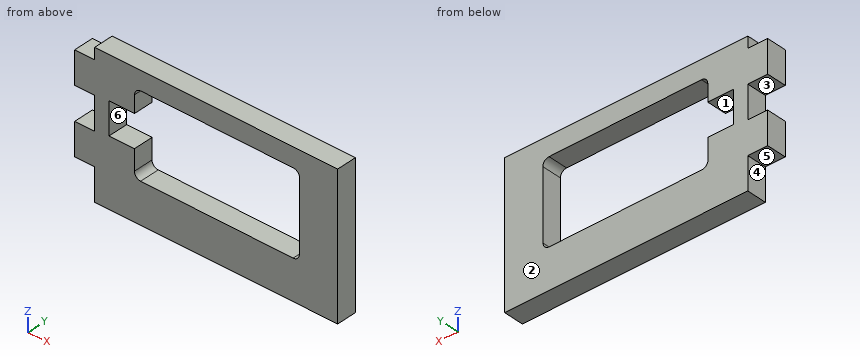
```python
from build123d import *

# Parameters (mm, degrees)
SKETCH1_W           = 127
SKETCH1_H           = 101.6
BOSS_EXTRUDE1_DEPTH = 4.800000052
CUT_EXTRUDE1_DEPTH  = 163.710171779
SKETCH4_W           = 127
SKETCH4_H           = 101.6
SKETCH4_W_2         = 63.302571571
SKETCH4_H_2         = 39.058596
CUT_EXTRUDE3_DEPTH  = 163.710171779
SKETCH5_W           = 4.800000052
SKETCH5_H           = 7.8117192
SKETCH5_H_2         = 7.874
SKETCH5_H_3         = 7.7494384
CUT_EXTRUDE4_DEPTH  = 133.639014141
SKETCH6_W           = 6.142649692
SKETCH6_H           = 7.722699729
CUT_EXTRUDE5_DEPTH  = 133.639014141
SKETCH7_W           = 58.502571519
SKETCH7_H           = 5.08
CUT_EXTRUDE6_DEPTH  = 133.639014141


with BuildPart() as part:
    # Sketch1 → Boss-Extrude1 (new body)
    with BuildSketch(Plane(origin=(0, 0, 0), x_dir=(1, 0, 0), z_dir=(0, 1, 0))):
        with Locations((63.5, 50.8)):
            Rectangle(SKETCH1_W, SKETCH1_H)
    extrude(amount=BOSS_EXTRUDE1_DEPTH)

    # Sketch3 → Cut-Extrude1 (cut, through all)
    with BuildSketch(Plane(origin=(0, 4.800000052, 0), x_dir=(1, 0, 0), z_dir=(0, 1, 0))):
        with BuildLine():
            Line((62.069935242, 45.315244869), (98.769812683, 45.432826029))
            ThreePointArc((98.769812683, 45.432826029), (99.829038472, 45.875546579), (100.264962787, 46.93758742))
            Line((100.264962787, 46.93758742), (100.211138047, 63.737569431))
            ThreePointArc((100.211138047, 63.737569431), (99.768417497, 64.79679522), (98.706376655, 65.232719535))
            Line((98.706376655, 65.232719535), (62.006499215, 65.115138375))
            ThreePointArc((62.006499215, 65.115138375), (60.947273426, 64.672417825), (60.51134911, 63.610376984))
            Line((60.51134911, 63.610376984), (60.565173851, 46.810394973))
            ThreePointArc((60.565173851, 46.810394973), (61.007894401, 45.751169184), (62.069935242, 45.315244869))
        make_face()
    extrude(amount=-CUT_EXTRUDE1_DEPTH, mode=Mode.SUBTRACT)

    # Sketch4 → Cut-Extrude3 (cut, through all)
    with BuildSketch(Plane.XZ):
        with Locations((63.5, -50.8)):
            Rectangle(SKETCH4_W, SKETCH4_H)
        with Locations((77.789401758, -55.255753861)):
            Rectangle(SKETCH4_W_2, SKETCH4_H_2, mode=Mode.SUBTRACT)
    extrude(amount=-CUT_EXTRUDE3_DEPTH, mode=Mode.SUBTRACT)

    # Sketch5 → Cut-Extrude4 (cut, through all)
    with BuildSketch(Plane.XZ):
        with Locations((48.538115998, -39.632315461)):
            Rectangle(SKETCH5_W, SKETCH5_H)
        with Locations((48.538115998, -55.286894261)):
            Rectangle(SKETCH5_W, SKETCH5_H_2)
        with Locations((48.538115998, -70.910332661)):
            Rectangle(SKETCH5_W, SKETCH5_H_3)
    extrude(amount=-CUT_EXTRUDE4_DEPTH, mode=Mode.SUBTRACT)

    # Sketch6 → Cut-Extrude5 (cut, through all)
    with BuildSketch(Plane.XZ):
        with Locations((57.480654221, -54.790150784)):
            Rectangle(SKETCH6_W, SKETCH6_H)
    extrude(amount=-CUT_EXTRUDE5_DEPTH, mode=Mode.SUBTRACT)

    # Sketch7 → Cut-Extrude6 (cut, through all)
    with BuildSketch(Plane(origin=(0, 4.800000052, 0), x_dir=(1, 0, 0), z_dir=(0, 1, 0))):
        with Locations((80.189401784, 38.266455861)):
            Rectangle(SKETCH7_W, SKETCH7_H)
    extrude(amount=-CUT_EXTRUDE6_DEPTH, mode=Mode.SUBTRACT)


solid = part.part
```
Geometry check sheet. Reference: the model listing, model coordinates, mm. Face numbers are marked on the shaded views. A direction names the side the tool comes from. Round coordinates to 2 decimals unless told otherwise and drop trailing zeros. Loops run counter-clockwise (first coordinate to the right, second up) from the corner with the lowest first, then second, coordinate; pieces in that order, holes last. Notation, with made-up numbers: M -13.75,-33 L 36.25,-33 A34 ccw 36.25,6 Z; hole C 28.5,-27 d11. An arc over 180 degrees is marked long. Return JSON: item names as keys, results as strings. Group by question number.
(1) Scan lines: line 1 along X through (y, z) = (0.35, -60); line 2 along X through (y, z) = (0.35, -49); line 3 along Z through (x, y) = (66, 4.15). Record each from-to range of solid material in increasing order. Write a range as [from, to].
(2) Section check C-C, the plane x = 74.5. Enter the section's corners in (y, z).
(3) Section check B-B, the plane z = -58. Enter the section's corners in (x, y).
(4) Go/stop test with a flat-tipped pin: pin 1 (1.4 mm diameter, centred on y = 3.5, z = -57.5, fed in from -X). Record where the tip stops, or that it passes through.
(5) Set-up check for the marked faces 1, 2 and 3: record each of +Z, -Z, +X, -X, +Y, -Y from which the full face is reachable in a straight line by a thin tool's end or side.
(6) Section check D-D, the plane z = -69. Enter the section's corners in (x, y), and give its area (3 significant figures).
(7) Section check A-A, the plane y = 3.25. Enter the section's corners in (x, z), and give its area (3 significant figures).
(8) Mould release check, pull along Z, two halves, no side actions. Record for the marked faces 4, 5 and 6: pulls with the +Z half, pulls with the -Z half, needs draft (parallel to the pull), parting line crosses it, or undercut.
Data:
{
 "1": {"line 1": "[46.14, 60.52], [100.22, 109.44]", "line 2": "[46.14, 60.56], [100.26, 109.44]", "line 3": "[-74.79, -65.13], [-45.33, -40.81]"},
 "2": {"outline": "M 0,-74.79 L 4.8,-74.79 L 4.8,-65.16 L 0,-65.16 Z; M 0,-45.36 L 4.8,-45.36 L 4.8,-40.81 L 0,-40.81 Z"},
 "3": {"outline": "M 50.94,0 L 54.41,0 L 54.41,4.8 L 50.94,4.8 Z; M 100.23,0 L 109.44,0 L 109.44,4.8 L 100.23,4.8 Z"},
 "4": {"pin 1": "x = 50.94"},
 "5": {"face 1": "+Y, -Y", "face 2": "+Z, -Z, +X, -X, +Y", "face 3": "-X, +Y, -Y"},
 "6": {"outline": "M 50.94,0 L 109.44,0 L 109.44,4.8 L 50.94,4.8 Z", "area": "281 mm²"},
 "7": {"outline": "M 46.14,-67.04 L 50.94,-67.04 L 50.94,-74.79 L 109.44,-74.79 L 109.44,-40.81 L 50.94,-40.81 L 50.94,-43.54 L 46.14,-43.54 L 46.14,-51.35 L 50.94,-51.35 L 50.94,-59.22 L 46.14,-59.22 Z; hole M 54.41,-58.65 L 60.53,-58.65 L 60.51,-63.61 A1.5 ccw 62.01,-65.12 L 98.71,-65.23 A1.5 ccw 100.21,-63.74 L 100.26,-46.94 A1.5 ccw 98.77,-45.43 L 62.07,-45.32 A1.5 ccw 60.57,-46.81 L 60.55,-50.93 L 54.41,-50.93 Z", "area": "1,230 mm²"},
 "8": {"face 4": "needs draft", "face 5": "pulls with the -Z half", "face 6": "undercut"}
}
